Answer from the drawing. Dimensions are ordinates in mm from the lowest x, y and z of the part. Coordinates: 2 decimals unless noted, no trailing zeros. Loops run counter-clockwise (first coordinate to the right, second up) from the corner with the lowest first, then second, coordinate; pieces in that order, holes last. Notation, with made-up numbers: (-23.75, 39) -> (-0.75, 39) arc R5 cw to (-0.75, 48) -> close; hole circle Ø10 at (-35.75, 32). An arc over 180 degrees is marked (long way). Use a Markdown table: item, result.
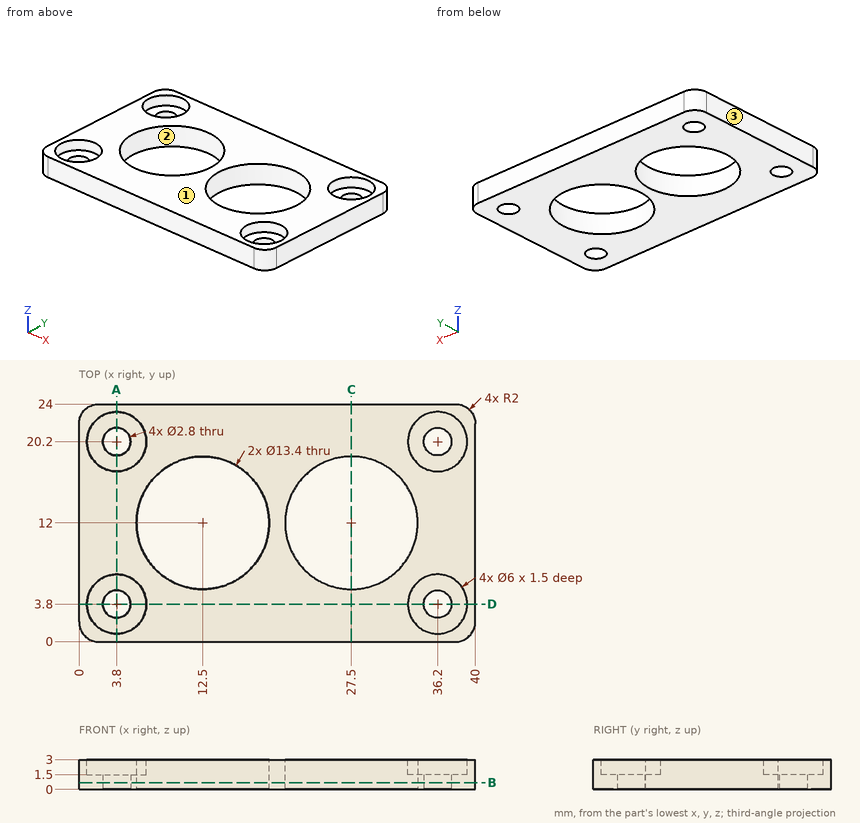
Q1. Section B-B on z = 0.7 is taken. Determine the outline of the cut face in (x, y).
Solved:
| item | result |
|---|---|
| outline | (0, 2) arc R2 ccw to (2, 0) -> (38, 0) arc R2 ccw to (40, 2) -> (40, 22) arc R2 ccw to (38, 24) -> (2, 24) arc R2 ccw to (0, 22) -> close; hole circle Ø2.8 at (3.8, 3.8); hole circle Ø2.8 at (3.8, 20.2); hole circle Ø13.4 at (12.5, 12); hole circle Ø13.4 at (27.5, 12); hole circle Ø2.8 at (36.2, 3.8); hole circle Ø2.8 at (36.2, 20.2) |
Q2. Section A-A on x = 3.8 is taken. Determine the outline of the cut face in (y, z), and give its area (3 significant figures).
Solved:
| item | result |
|---|---|
| outline | (0, 0) -> (2.4, 0) -> (2.4, 1.5) -> (0.8, 1.5) -> (0.8, 3) -> (0, 3) -> close; (5.2, 0) -> (18.8, 0) -> (18.8, 1.5) -> (17.2, 1.5) -> (17.2, 3) -> (6.8, 3) -> (6.8, 1.5) -> (5.2, 1.5) -> close; (21.6, 0) -> (24, 0) -> (24, 3) -> (23.2, 3) -> (23.2, 1.5) -> (21.6, 1.5) -> close |
| area | 45.6 mm² |
Q3. Consider line 1 (Y direction, x = 3.8, z = 2.6); line 2 (X direction, y = 4, z = 2.3); line 3 (Y direction, x = 3.8, z = 1.05). Determine where each line is inside the solid, lowest interval first. Write a range as [from, to].
Solved:
| item | result |
|---|---|
| line 1 | [0, 0.8], [6.8, 17.2], [23.2, 24] |
| line 2 | [0, 0.81], [6.79, 33.21], [39.19, 40] |
| line 3 | [0, 2.4], [5.2, 18.8], [21.6, 24] |
Q4. Given pin 1 Ø4.5 at (x, y) = (36.2, 3.8) entering from +Z, flat-ended and moving along its own axis, determine where the tip first touches the part or whether it passes through.
Solved:
| item | result |
|---|---|
| pin 1 | z = 1.5 |
Q5. Section D-D on y = 3.8 is taken. Determine the outline of the cut face in (x, z).
Solved:
| item | result |
|---|---|
| outline | (0, 0) -> (2.4, 0) -> (2.4, 1.5) -> (0.8, 1.5) -> (0.8, 3) -> (0, 3) -> close; (5.2, 0) -> (34.8, 0) -> (34.8, 1.5) -> (33.2, 1.5) -> (33.2, 3) -> (6.8, 3) -> (6.8, 1.5) -> (5.2, 1.5) -> close; (37.6, 0) -> (40, 0) -> (40, 3) -> (39.2, 3) -> (39.2, 1.5) -> (37.6, 1.5) -> close |
Q6. Section C-C on x = 27.5 is taken. Determine the outline of the cut face in (y, z), and give its area (3 significant figures).
Solved:
| item | result |
|---|---|
| outline | (0, 0) -> (5.3, 0) -> (5.3, 3) -> (0, 3) -> close; (18.7, 0) -> (24, 0) -> (24, 3) -> (18.7, 3) -> close |
| area | 31.8 mm² |
Q7. Determine the mould class of the marked faces 1, 2 and 3 for opening direction X: pulls with the +X half, pulls with the -X half, needs draft (parallel to the pull), parting line crosses it, or undercut.
Solved:
| item | result |
|---|---|
| face 1 | needs draft |
| face 2 | undercut |
| face 3 | pulls with the -X half |
